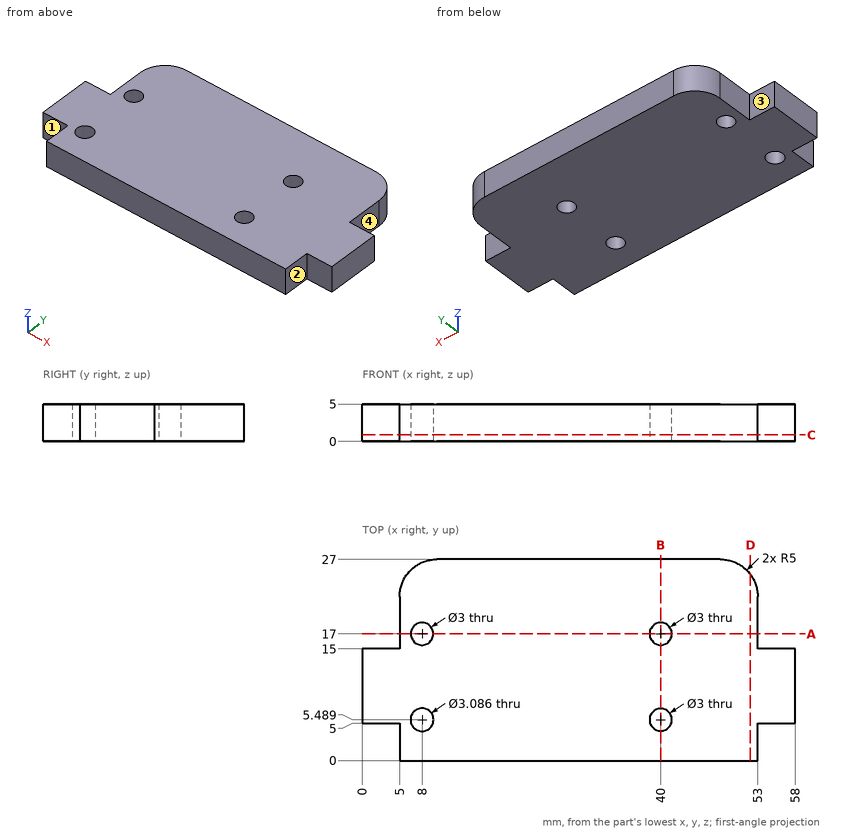
Design review of the part shown in the three views and the two pictorial views. Dimensions are in mm from the part's minimum x, y and z. A direction names the side the tool comes from. Round coordinates to 2 decimals unless told otherwise and drop trailing zeros. Loops run counter-clockwise (first coordinate to the right, second up) from the corner with the lowest first, then second, coordinate; pieces in that order, holes last. Notation, with made-up numbers: M 54.5,55 L 82.5,55 A22 ccw 82.5,67 Z; hole C 3.25,-20 d9. An arc over 180 degrees is marked long. Put each result on its own line as item: value.
Q1. Machinability: for the marked faces 1, 2, 3 and 4, which of the approach directions +Z, -Z, +X, -X, +Y, -Y give a long, thin tool a straight path to every point of the face, cutting with its end or side? Answer none if there is none.
Result set:
face 1: +Z, -Z, -X, -Y
face 2: +Z, -Z, +X, -Y
face 3: +Z, -Z, -X, +Y
face 4: +Z, -Z, +X, +Y
Q2. Consider section C-C, the plane z = 0.85. Give the boundary of the cut face in (x, y).
Result set:
outline: M 0,5 L 5,5 L 5,0 L 53,0 L 53,5 L 58,5 L 58,15 L 53,15 L 53,22 A5 ccw 48,27 L 10,27 A5 ccw 5,22 L 5,15 L 0,15 Z; hole C 8,5.49 d3.09; hole C 8,17 d3; hole C 40,5.49 d3; hole C 40,17 d3
Q3. Consider section B-B, the plane x = 40. Give the boundary of the cut face in (y, z), then the cut area to 3 significant figures.
Result set:
outline: M 0,0 L 3.99,0 L 3.99,5 L 0,5 Z; M 6.99,0 L 15.5,0 L 15.5,5 L 6.99,5 Z; M 18.5,0 L 27,0 L 27,5 L 18.5,5 Z
area: 105 mm²
Q4. Consider section A-A, the plane y = 17. Give the boundary of the cut face in (x, z).
Result set:
outline: M 5,0 L 6.5,0 L 6.5,5 L 5,5 Z; M 9.5,0 L 38.5,0 L 38.5,5 L 9.5,5 Z; M 41.5,0 L 53,0 L 53,5 L 41.5,5 Z
Q5. Consider section D-D, the plane x = 52. Give the boundary of the cut face in (y, z).
Result set:
outline: M 0,0 L 25,0 L 25,5 L 0,5 Z
Q6. For pin 1 (1.5 mm diameter, centred on y = 3.5, z = 3.5, fed in from +X); pin 2 (2.5 mm diameter, centred on x = 2, z = 2.5, fed in from -Y), all flat-tipped, find the tip position at first contact; note any pin that passes through.
Result set:
pin 1: stops at x = 53
pin 2: stops at y = 5
Q7. To check wall thickness, follow L1, parallel to Y at x = 40, z = 1.4; L2, parallel to Y at x = 8, z = 1.35 (1 decimal); L3, parallel to X at y = 16, z = 1.1. State the ranges of each line that lie inside material, in increasing order.
Result set:
L1: y = 0 to 3.99, 6.99 to 15.5, 18.5 to 27
L2: y = 0 to 3.9, 7 to 15.5, 18.5 to 26.6
L3: x = 5 to 6.88, 9.12 to 38.88, 41.12 to 53
